Could you check a few things on this model? Use its own coordinates, in mm. Round coordinates to 2 decimals unless told otherwise and drop trailing zeros. Loops run counter-clockwise (first coordinate to the right, second up) from the corner with the lowest first, then second, coordinate; pieces in that order, holes last. Notation, with made-up numbers: M -38,55 L 2,55 A17 ccw 2,65 Z; hole C 75.5,59 d8. An arc over 180 degrees is marked long. One line per item, written item: value. Start each with the question number.
Q1. Imagine slicing it at B-B (y = 57.5). Please give me the cut outline in (x, z).
Q2. I'm going to push flat-ended pins straight in: pin 1 Ø1 at (x, y) = (-21, 29) entering from -Z; pin 2 Ø1.5 at (x, y) = (-23, 62) entering from -Z; pin 3 Ø2.5 at (x, z) = (-22, 2.5) entering from +Y; pin 4 Ø1.5 at (x, z) = (-24, 2.5) entering from -Y. Where does each tip first touch, or does it pass through?
Q3. Imagine slicing it at A-A (x = -24). Please give me the cut outline in (y, z).
Q4. Please list where these lines run through material, in increasing order: line 1 along Y through (x, z) = (-23.8, 3); line 2 along Z through (x, y) = (-23.05, -53).
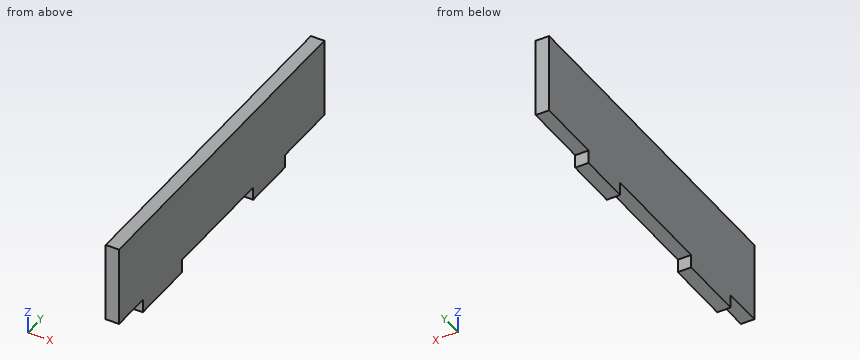
from build123d import *

# Parameters (mm, degrees)
SKETCH1_W             = 5
SKETCH1_H             = 20
BOSS_EXTRUDE1_DEPTH   = 5
SKETCH1_H_2           = 25
BOSS_EXTRUDE1_2_DEPTH = 5
SKETCH2_W             = 5
SKETCH2_H             = 130
BOSS_EXTRUDE2_DEPTH   = 30


with BuildPart() as part:
    # Sketch1 → Boss-Extrude1 (new body)
    with BuildSketch(Plane.XY):
        with Locations((-22.883589858, 35.86307718)):
            Rectangle(SKETCH1_W, SKETCH1_H)
    extrude(amount=BOSS_EXTRUDE1_DEPTH)



with BuildPart() as body_2:
    # Sketch1 → Boss-Extrude1 2 (new body)
    with BuildSketch(Plane.XY):
        with Locations((-22.883589858, -31.63692282)):
            Rectangle(SKETCH1_W, SKETCH1_H_2)
    extrude(amount=BOSS_EXTRUDE1_2_DEPTH)


with BuildPart() as part_1:
    add(part.part)

    add(body_2.part)  # Boss-Extrude2 merges body 2
    # Sketch2 → Boss-Extrude2 (add)
    with BuildSketch(Plane.XY.offset(5)):
        with Locations((-22.883589858, 5.86307718)):
            Rectangle(SKETCH2_W, SKETCH2_H)
    extrude(amount=BOSS_EXTRUDE2_DEPTH)


solid = part_1.part
Report:
1. outline: M -25.38,5 L -20.38,5 L -20.38,35 L -25.38,35 Z
2. pin 1: stops at z = 0
2. pin 2: stops at z = 5
2. pin 3: stops at y = 45.86
2. pin 4: stops at y = -44.14
3. outline: M -59.14,5 L -44.14,5 L -44.14,0 L -19.14,0 L -19.14,5 L 25.86,5 L 25.86,0 L 45.86,0 L 45.86,5 L 70.86,5 L 70.86,35 L -59.14,35 Z
4. line 1: y = -44.14 to -19.14, 25.86 to 45.86
4. line 2: z = 5 to 35
